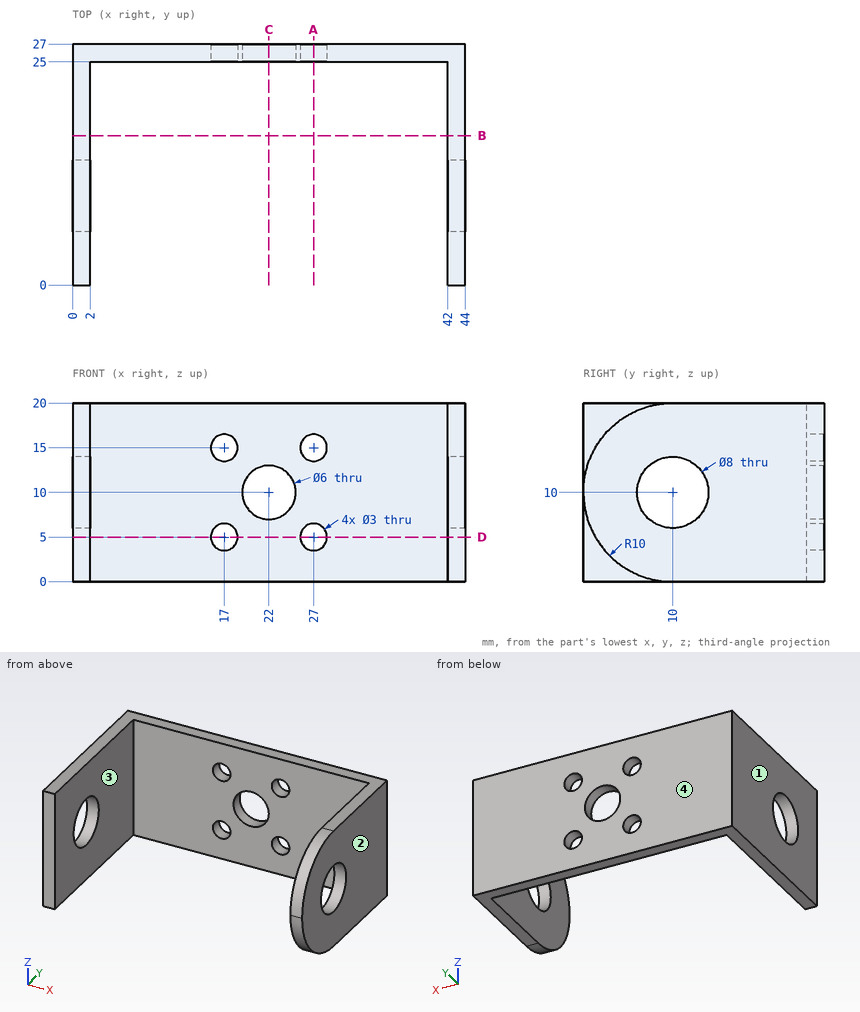
Job drawing, mm, ordinate dimensions from the low corner. One solid piece. Round coordinates to 2 decimals unless told otherwise and drop trailing zeros. Write each loop counter-clockwise with the first axis right and the second up, starting at its lowest first coordinate (ties: lowest second). Pieces come first, ordered by that corner, then holes.
1) Band-saw the part on A-A, the plane x = 27. List the corners of the cut face in (y, z), and give its area (3 significant figures).
2) Band-saw the part on C-C, the plane x = 22. List the corners of the cut face in (y, z), and give its area (3 significant figures).
3) Pin check, flat tip, straight feed: pin 1 (3 mm diameter, centred on x = 25.5, z = 14, fed in from -Y). Stop position of the tip, or through.
4) Drill centre lines: probe 1 along Z at (x, y) = (17, 26.35); probe 2 along X at (y, z) = (13, 18.5); probe 3 along Z at (x, y) = (1, 10). Where is each one in solid material? Low to high.
5) Mould opens along X. For the marked faces 1, 2, 3 and 4 say: +X half, -X half, draft (parallel to the pull), parting line (faces both ways), or undercut.
6) Band-saw the part on B-B, the plane y = 16.75. List the corners of the cut face in (x, z), and give its area (3 significant figures).
7) Band-saw the part on D-D, the plane z = 5. List the corners of the cut face in (x, y).
Ans:
1. outline: (25, 0) - (27, 0) - (27, 3.5) - (25, 3.5) - close; (25, 6.5) - (27, 6.5) - (27, 13.5) - (25, 13.5) - close; (25, 16.5) - (27, 16.5) - (27, 20) - (25, 20) - close
1. area: 28.0 mm2
2. outline: (25, 0) - (27, 0) - (27, 7) - (25, 7) - close; (25, 13) - (27, 13) - (27, 20) - (25, 20) - close
2. area: 28.0 mm2
3. pin 1: stops at y = 25
4. probe 1: z = 0 to 3.5, 6.5 to 13.5, 16.5 to 20
4. probe 2: x = 0 to 2, 42 to 44
4. probe 3: z = 0 to 6, 14 to 20
5. face 1: -X half
5. face 2: +X half
5. face 3: undercut
5. face 4: draft
6. outline: (0, 0) - (2, 0) - (2, 20) - (0, 20) - close; (42, 0) - (44, 0) - (44, 20) - (42, 20) - close
6. area: 80.0 mm2
7. outline: (0, 0) - (2, 0) - (2, 25) - (15.5, 25) - (15.5, 27) - (0, 27) - close; (18.5, 25) - (25.5, 25) - (25.5, 27) - (18.5, 27) - close; (28.5, 25) - (42, 25) - (42, 1.34) - (44, 1.34) - (44, 27) - (28.5, 27) - close
